from build123d import *

# Parameters (mm, degrees)
F3_DEPTH = 3.175
F4_R     = 2.413
F5_DEPTH = 5.55625


with BuildPart() as f1:
    # F0 (on Front) → F1 (revolve)
    with BuildSketch(Plane.XZ):
        with BuildLine():
            Line((0, 0), (0, 92.86875))
            Line((0, 92.86875), (0, 95.43415))
            ThreePointArc((0, 95.43415), (-2.626821, 94.749192), (-4.5847, 92.86875))
            Line((-4.5847, 92.86875), (-2.413, 92.86875))
            Line((-2.413, 92.86875), (-2.413, 0))
            Line((-2.413, 0), (0, 0))
        make_face()
    revolve(axis=Axis((0, 0, 46.434375), (0, 0, -1)))

    # F2 (on face) → F3 (join)
    with BuildSketch(Plane(origin=(0, 0, 0), x_dir=(1, 0, 0), z_dir=(0, 0, -1))):
        Polygon((2.749631, 4.7625), (-2.749631, 4.7625), (-5.499261, 0), (-2.749631, -4.7625), (2.749631, -4.7625), (5.499261, 0), align=None)
    extrude(amount=F3_DEPTH)

    # F4 (on face) → F5 (join)
    with BuildSketch(Plane(origin=(0, 0, -3.175), x_dir=(1, 0, 0), z_dir=(0, 0, -1))):
        Circle(F4_R)
    extrude(amount=F5_DEPTH)


solid = f1.part
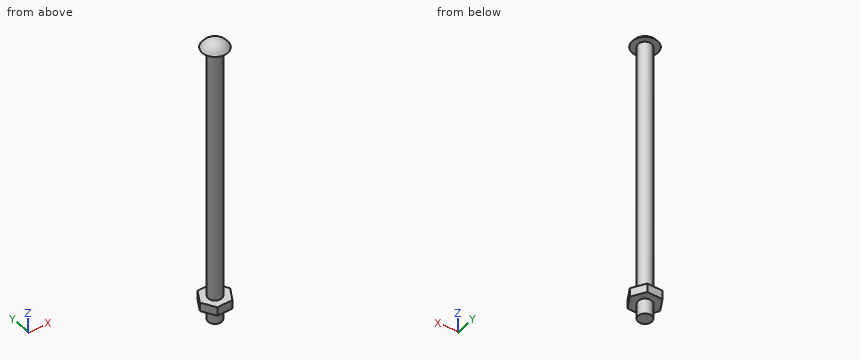
Model file for the job. Use its own axes, mm. Give positions to 0.01 mm unless a question says otherwise; leave off trailing zeros. Loops run counter-clockwise (first coordinate to the right, second up) from the corner with the lowest first, then second, coordinate; pieces in that order, holes last.
Item 1: Drop flat-ended pins along their axis: P1, Ø1.5, axis at y = 1, z = 42.5, coming from the -X side; P2, Ø5, axis at x = 2.5, y = 2, coming from the -Z side; P3, Ø2, axis at x = -0.5, z = 70.5, coming from the +Y side. Give the stop position or say it passes through.
Check values:
P1: stops at x = -2.4
P2: stops at z = -8.73
P3: stops at y = 2.41
Item 2: Slice it at A-A (z = 31.5). Write the cut outline in (x, y), plus the area to 3 significant figures.
Check values:
outline: circle Ø4.83 at (0, 0)
area: 18.3 mm2
Item 3: Drill centre lines: line 1 along Z through (x, y) = (3.25, -1) (3 decimals); line 2 along Z through (x, y) = (-5, -0.5) (3 decimals); line 3 along Z through (x, y) = (1.5, 2.75) (3 decimals). Where is each one in solid material? Low to high.
Check values:
line 1: z = -3.175 to 0, 92.869 to 94.223
line 2: z = -3.175 to 0
line 3: z = -3.175 to 0, 92.869 to 94.428
